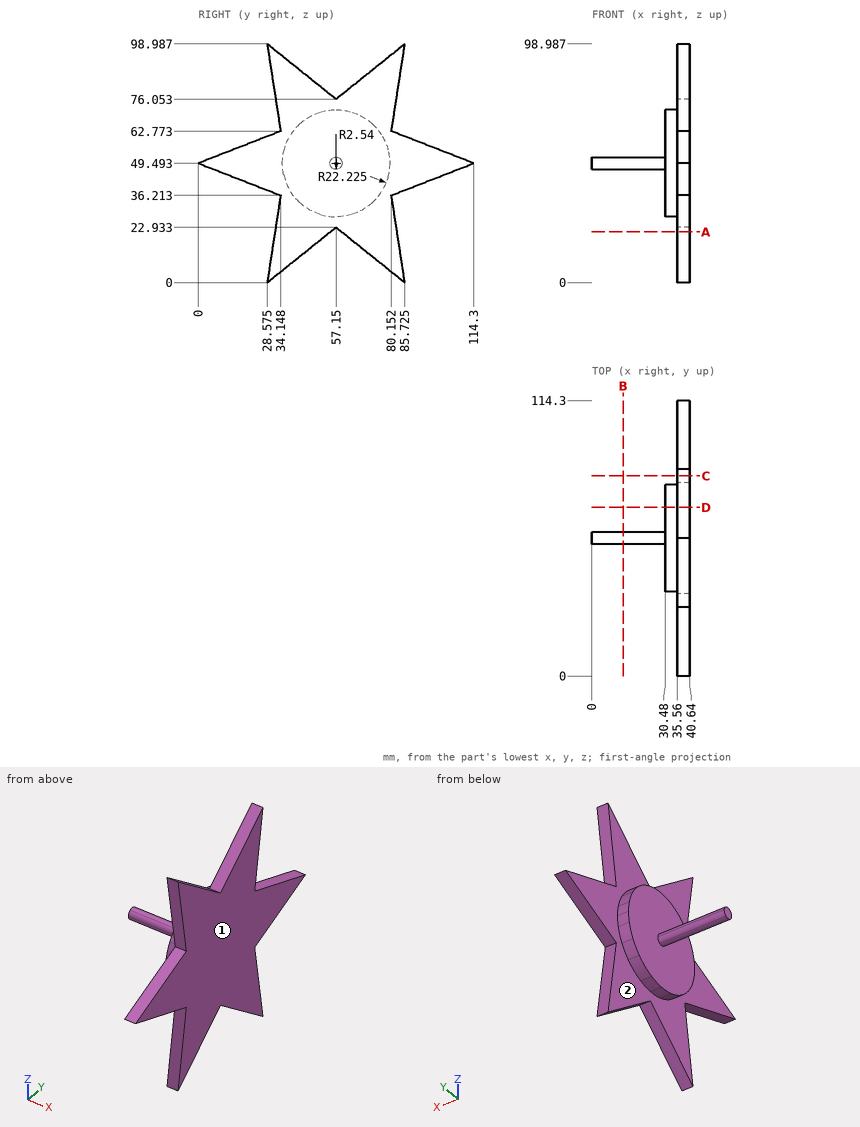
The drawing under review shows one solid part. Ordinate dimensions are in mm from its lowest x, y, z. A direction names the side the tool comes from. Round coordinates to 2 decimals unless told otherwise and drop trailing zeros. Order: outer loops, then holes, each group sorted by start corner. A loop starts at its lowest first (then second) coordinate and runs counter-clockwise, first axis right, second up. Notation, with made-up numbers: (83.25, 44) -> (93.25, 44) arc R28 ccw to (93.25, 64) -> close; hole circle Ø2 at (8, 79). An arc over 180 degrees is marked (long way). Return JSON: item names as keys, results as strings.
1. Take a section at C-C (y = 83). Write out the cut boundary in (x, z) (1 decimal).
Answer block:
{"outline": "(35.6, 2.2) -> (40.6, 2.2) -> (40.6, 17.7) -> (35.6, 17.7) -> close; (35.6, 37.3) -> (40.6, 37.3) -> (40.6, 61.7) -> (35.6, 61.7) -> close; (35.6, 81.3) -> (40.6, 81.3) -> (40.6, 96.8) -> (35.6, 96.8) -> close"}
2. Take a section at A-A (z = 21). Write out the cut boundary in (x, y).
Answer block:
{"outline": "(35.56, 31.81) -> (40.64, 31.81) -> (40.64, 54.74) -> (35.56, 54.74) -> close; (35.56, 59.56) -> (40.64, 59.56) -> (40.64, 82.49) -> (35.56, 82.49) -> close"}
3. Insertion check: P1, Ø13.5, axis at y = 50.5, z = 46.5, coming from the -X side; P2, Ø10, axis at x = 14.5, z = 51, coming from the +Y side; P3, Ø12, axis at x = 36, y = 38.5, coming from the +Z side; P4, Ø8, axis at y = 34, z = 35.5, coming from the -X side. Each pin has a flat end and moves straight along its axis. Give the tip position at first contact, or say it passes through.
Answer block:
{"P1": "stops at x = 0", "P2": "stops at y = 59.69", "P3": "stops at z = 95.84", "P4": "stops at x = 35.56"}
4. Take a section at D-D (y = 70). Write out the cut boundary in (x, z).
Answer block:
{"outline": "(30.48, 31.36) -> (35.56, 31.36) -> (35.56, 12.62) -> (40.64, 12.62) -> (40.64, 86.37) -> (35.56, 86.37) -> (35.56, 67.63) -> (30.48, 67.63) -> close"}
5. For L1, parallel to X at y = 64.5, z = 60; L2, parallel to X at y = 43.5, z = 20; L3, parallel to Z at x = 39.5, y = 49 (1 decimal), list the stretches that pass through material, from the lowest coordinate up. Write a range as [from, to].
Answer block:
{"L1": "x = [30.48, 40.64]", "L2": "x = [35.56, 40.64]", "L3": "z = [16.4, 82.6]"}
6. For the marked faces 1 and 2, list the 3-axis set-ups (+Z, -Z, +X, -X, +Y, -Y) from which the entire face can be reached by the end or side of a thin tool; tool diameter is ignored.
Answer block:
{"face 1": "+Z, -Z, +X, +Y, -Y", "face 2": "-X"}
7. Take a section at B-B (x = 13). Write out the cut boundary in (y, z), then the cut area to 3 significant figures.
Answer block:
{"outline": "circle Ø5.08 at (57.15, 49.49)", "area": "20.3 mm²"}
